Verification items for the finished model (mm, model axes). A direction names the side the tool comes from. Coordinates: 2 decimals unless noted, no trailing zeros. Loops run counter-clockwise (first coordinate to the right, second up) from the corner with the lowest first, then second, coordinate; pieces in that order, holes last. Notation, with made-up numbers: (48.25, -24.5) - (65.25, -24.5) arc R19 cw to (65.25, -18.5) - close; hole circle Ø10 at (1, 0.5). An arc over 180 degrees is marked (long way). One line per item, written item: value. Start each with the question number.
(1) Draft check along X on faces 5 (the face through (87, 3, 103.5)), 6 (the face through (-121.539, 3, -63)), 7 (the face through (-83, 3, -94.5)). Enter one of: +X half, -X half, draft (parallel to the pull), parting line (faces both ways), or undercut.
(2) Section check A-A (x = -71). Record the boundary of the cut face in (y, z), plus the area to 3 significant figures.
(3) Gauge pin test, flat ends, axial feed: P1, Ø1.8, axis at y = 2, z = -61, coming from the -X side; P2, Ø2, axis at x = -88.5, y = 3, coming from the +Z side. Record the tip position at first contact, or that the pin passes through.
(4) Set-up check for faces 1 (the face through (42.461, 3, -97)), 2 (the face through (96.461, 3, -80)), 3 (the face through (-82, 3, 97.5)), 4 (the face through (-121.539, 3, 29)): record each of +Z, -Z, +X, -X, +Y, -Y from which the full face is reachable in a straight line by a thin tool's end or side.
(5) Section check C-C (z = -68). Record the boundary of the cut face in (x, y).
(6) Section check B-B (y = 3.9). Count the separate pieces of the cut face and the enclosed holes in it, plus the area to 3 significant figures.
(7) Thickness scan on probe 1 along X at (y, z) = (2.1, 23); probe 2 along Z at (x, y) = (68.5, 5.25); probe 3 along X at (y, z) = (3.75, 42). Record the ranges inside material, lowest first. Write a range as [from, to].
Autodesk Inventor part; units mm, degrees
ref_plane "YZ Plane" through (0, 0, 0) normal (1, 0, 0) x (0, 1, 0)
ref_plane "XZ Plane" through (0, 0, 0) normal (0, 1, 0) x (-1, 0, 0)
ref_plane "XY Plane" through (0, 0, 0) normal (0, 0, 1) x (1, 0, 0)
sketch "Эскиз1" plane through (0, 0, 0) normal (0, 1, 0) x (-1, 0, 0)
  line L0 (127.5386, 103.5005) -> (-102.4614, 103.5005)
  line L1 (-102.4614, 103.5005) -> (-102.4614, -100.4995)
  line L2 (-102.4614, -100.4995) -> (127.5386, -100.4995)
  line L3 (127.5386, -100.4995) -> (127.5386, 103.5005)
  line L4 (127.5386, -100.4995) -> (97.5386, -100.4995)
  line L5 (97.5386, -100.4995) -> (97.5386, -94.4995)
  line L6 (97.5386, -94.4995) -> (127.5386, -94.4995)
  line L7 (127.5386, -94.4995) -> (127.5386, -100.4995)
  line L8 (97.5386, -94.4995) -> (67.5386, -94.4995)
  line L9 (67.5386, -94.4995) -> (67.5386, -100.4995)
  line L10 (67.5386, -100.4995) -> (97.5386, -100.4995)
  line L11 (97.5386, -100.4995) -> (97.5386, -94.4995)
  line L12 (6.9803, -100.4995) -> (67.5386, -100.4995)
  line L13 (67.5386, -100.4995) -> (67.5386, -94.4995)
  line L14 (-42.4614, -94.4995) -> (-42.4614, -100.4995)
  line L15 (-42.4614, -100.4995) -> (-2.4614, -100.4995)
  line L16 (-42.4614, -94.4995) -> (-72.4614, -94.4995)
  line L17 (-72.4614, -94.4995) -> (-72.4614, -100.4995)
  line L18 (-72.4614, -100.4995) -> (-42.4614, -100.4995)
  line L19 (-42.4614, -100.4995) -> (-42.4614, -94.4995)
  line L20 (-72.4614, -94.4995) -> (-102.4614, -94.4995)
  line L21 (-102.4614, -94.4995) -> (-102.4614, -100.4995)
  line L22 (-102.4614, -100.4995) -> (-72.4614, -100.4995)
  line L23 (-72.4614, -100.4995) -> (-72.4614, -94.4995)
  line L24 (-42.4614, -94.4995) -> (-2.4614, -94.4995)
  line L25 (-2.4614, -94.4995) -> (-2.4614, -100.4995)
  line L26 (-2.4614, -100.4995) -> (-42.4614, -100.4995)
  line L27 (-42.4614, -100.4995) -> (-42.4614, -94.4995)
  line L28 (-2.4614, -100.4995) -> (27.5386, -100.4995)
  line L29 (27.5386, -100.4995) -> (27.5386, -94.4995)
  line L30 (27.5386, -94.4995) -> (-2.4614, -94.4995)
  line L31 (-2.4614, -94.4995) -> (-2.4614, -100.4995)
  line L32 (67.5386, -94.4995) -> (27.5386, -94.4995)
  line L33 (27.5386, -94.4995) -> (27.5386, -100.4995)
  line L34 (27.5386, -100.4995) -> (67.5386, -100.4995)
  line L35 (67.5386, -100.4995) -> (67.5386, -94.4995)
  line L36 (-102.4614, 97.5005) -> (127.5386, 97.5005)
  line L37 (127.5386, 97.5005) -> (97.5386, 97.5005)
  line L38 (97.5386, 97.5005) -> (97.5386, 103.5005)
  line L39 (97.5386, 103.5005) -> (127.5386, 103.5005)
  line L40 (127.5386, 103.5005) -> (127.5386, 97.5005)
  line L41 (97.5386, 103.5005) -> (67.5386, 103.5005)
  line L42 (67.5386, 103.5005) -> (67.5386, 97.5005)
  line L43 (67.5386, 97.5005) -> (97.5386, 97.5005)
  line L44 (97.5386, 97.5005) -> (97.5386, 103.5005)
  line L45 (6.9803, 97.5005) -> (67.5386, 97.5005)
  line L46 (67.5386, 97.5005) -> (67.5386, 103.5005)
  line L47 (-42.4614, 103.5005) -> (-42.4614, 97.5005)
  line L48 (-42.4614, 97.5005) -> (-2.4614, 97.5005)
  line L49 (-42.4614, 103.5005) -> (-72.4614, 103.5005)
  line L50 (-72.4614, 103.5005) -> (-72.4614, 97.5005)
  line L51 (-72.4614, 97.5005) -> (-42.4614, 97.5005)
  line L52 (-42.4614, 97.5005) -> (-42.4614, 103.5005)
  line L53 (-72.4614, 103.5005) -> (-102.4614, 103.5005)
  line L54 (-102.4614, 103.5005) -> (-102.4614, 97.5005)
  line L55 (-102.4614, 97.5005) -> (-72.4614, 97.5005)
  line L56 (-72.4614, 97.5005) -> (-72.4614, 103.5005)
  line L57 (-42.4614, 103.5005) -> (-2.4614, 103.5005)
  line L58 (-2.4614, 103.5005) -> (-2.4614, 97.5005)
  line L59 (-2.4614, 97.5005) -> (-42.4614, 97.5005)
  line L60 (-42.4614, 97.5005) -> (-42.4614, 103.5005)
  line L61 (-2.4614, 97.5005) -> (27.5386, 97.5005)
  line L62 (27.5386, 97.5005) -> (27.5386, 103.5005)
  line L63 (27.5386, 103.5005) -> (-2.4614, 103.5005)
  line L64 (-2.4614, 103.5005) -> (-2.4614, 97.5005)
  line L65 (67.5386, 103.5005) -> (27.5386, 103.5005)
  line L66 (27.5386, 103.5005) -> (27.5386, 97.5005)
  line L67 (27.5386, 97.5005) -> (67.5386, 97.5005)
  line L68 (67.5386, 97.5005) -> (67.5386, 103.5005)
  line L69 (-102.4614, 63.5005) -> (-96.4614, 63.5005)
  line L70 (-96.4614, 63.5005) -> (-96.4614, 33.5005)
  line L71 (-96.4614, 33.5005) -> (-102.4614, 33.5005)
  line L72 (-102.4614, 33.5005) -> (-102.4614, 63.5005)
  line L73 (-102.4614, -30.4995) -> (-96.4614, -30.4995)
  line L74 (-96.4614, -30.4995) -> (-96.4614, -60.4995)
  line L75 (-96.4614, -60.4995) -> (-102.4614, -60.4995)
  line L76 (-102.4614, -60.4995) -> (-102.4614, -30.4995)
  line L77 (127.5386, 63.5005) -> (121.5386, 63.5005)
  line L78 (121.5386, 33.5005) -> (127.5386, 33.5005)
  line L79 (127.5386, 33.5005) -> (127.5386, 63.5005)
  line L80 (127.5386, -50.4995) -> (93.2543, -50.4995)
  line L81 (121.5386, -60.4995) -> (127.5386, -60.4995)
  line L82 (127.5386, -60.4995) -> (127.5386, -50.4995)
  line L83 (-102.4614, 88.5005) -> (-96.4614, 88.5005)
  line L84 (-96.4614, 88.5005) -> (-96.4614, 78.5005)
  line L85 (-96.4614, 78.5005) -> (-102.4614, 78.5005)
  line L86 (-102.4614, 78.5005) -> (-102.4614, 88.5005)
  line L87 (-102.4614, -75.4995) -> (-96.4614, -75.4995)
  line L88 (-96.4614, -75.4995) -> (-96.4614, -85.4995)
  line L89 (-96.4614, -85.4995) -> (-102.4614, -85.4995)
  line L90 (-102.4614, -85.4995) -> (-102.4614, -75.4995)
  line L91 (127.5386, 73.5005) -> (121.5386, 73.5005)
  line L92 (121.5386, 73.5005) -> (121.5386, 58.5005)
  line L93 (121.5386, 58.5005) -> (127.5386, 58.5005)
  line L94 (127.5386, 58.5005) -> (127.5386, 73.5005)
  line L95 (127.5386, -55.4995) -> (121.5386, -55.4995)
  line L96 (121.5386, -55.4995) -> (121.5386, -70.4995)
  line L97 (121.5386, -70.4995) -> (127.5386, -70.4995)
  line L98 (127.5386, -70.4995) -> (127.5386, -55.4995)
  line L99 (127.5386, 38.5005) -> (121.5386, 38.5005)
  line L100 (121.5386, 38.5005) -> (121.5386, 18.5005)
  line L101 (121.5386, 18.5005) -> (127.5386, 18.5005)
  line L102 (127.5386, 18.5005) -> (127.5386, 38.5005)
  line L103 (127.5386, -15.4995) -> (121.5386, -15.4995)
  line L104 (121.5386, -15.4995) -> (121.5386, -35.4995)
  line L105 (121.5386, -35.4995) -> (127.5386, -35.4995)
  line L106 (127.5386, -35.4995) -> (127.5386, -15.4995)
  point P0 (0, 0)
  point P1 (-42.4614, -97.4995)
  point P2 (67.5386, -97.4995)
  point P3 (-42.4614, 100.5005)
  point P4 (67.5386, 100.5005)
  point P5 (-99.4614, -60.4995)
  point P6 (97.5386, 103.5005)
  point P7 (67.5386, 103.5005)
  point P8 (27.5386, 103.5005)
  point P9 (27.5386, 97.5005)
  point P10 (-2.4614, 103.5005)
  point P11 (-42.4614, 103.5005)
  point P12 (-102.4614, 33.5005)
  point P13 (-2.4614, -100.4995)
  point P14 (124.5386, 63.5005)
  point P15 (124.5386, -60.4995)
  point P16 (127.5386, 33.5005)
  point P17 (127.5386, 97.5005)
  point P18 (-102.4614, 97.5005)
  point P19 (97.5386, 97.5005)
  point P20 (27.5386, 103.5005)
  point P21 (-2.4614, 97.5005)
  point P22 (27.5386, 97.5005)
  point P23 (-2.4614, -100.4995)
  point P24 (-99.4614, 88.5005)
  point P25 (-99.4614, 78.5005)
  point P26 (-99.4614, 63.5005)
  point P27 (-99.4614, -75.4995)
  point P28 (124.5386, 73.5005)
  point P29 (124.5386, 58.5005)
  point P30 (124.5386, -70.4995)
  point P31 (124.5386, 38.5005)
  point P32 (124.5386, -55.4995)
  point P33 (124.5386, -35.4995)
  dimension "d0" = 230
  dimension "d1" = 204
  dimension "d2" = 6
  dimension "d3" = 30
  dimension "d4" = 30
  dimension "d5" = 30
  dimension "d6" = 30
  dimension "d8" = 40
  dimension "d10" = 40
  dimension "d11" = 230
  dimension "d13" = 6
  dimension "d14" = 30
  dimension "d15" = 30
  dimension "d16" = 30
  dimension "d17" = 30
  dimension "d18" = 40
  dimension "d19" = 40
  dimension "d20" = 40
  dimension "d21" = 30
  dimension "d22" = 40
  dimension "d23" = 30
  dimension "d24" = 6
  dimension "d27" = 6
  dimension "d28" = 40
  dimension "d29" = 40
  dimension "d30" = 30
  dimension "d31" = 30
  dimension "d84" = 10
  dimension "d85" = 15
  dimension "d86" = 15
  dimension "d87" = 10
  dimension "d88" = 6
  dimension "d89" = 6
  dimension "d90" = 15
  dimension "d91" = 15
  dimension "d92" = 30
  dimension "d93" = 30
  dimension "d94" = 20
  dimension "d95" = 20
  dimension "d96" = 20
  dimension "d97" = 20
extrude "Выдавливание1" add sketch "Эскиз1" along normal blind 6 contours L3 L36 L38 L0 | L3 L91 L92 L93 L99 L100 L101 L103 L104 L105 L95 L96 L97 L6 L8 L32 L30 L24 L16 L20 L1 L89 L88 L87 L75 L74 L73 L71 L70 L69 L85 L84 L83 L36 | L42 L36 L62 L0 | L58 L36 L47 L0 | L50 L36 L1 L0 | L3 L2 L5 L6 | L9 L2 L29 L32 | L20 L17 L2 L1 | L25 L2 L14 L24
sketch "Эскиз2" plane through (0, 6, 0) normal (0, 1, 0) x (1, 0, 0)
  point P0 (0, 0)
sketch "Эскиз5" plane through (0, 0, 0) normal (0, -1, 0) x (1, 0, 0)
  circle A0 centre (22.4614, 100.5005) radius 1.5
  circle A1 centre (-47.5386, 100.5005) radius 1.5
  circle A2 centre (-47.5386, -97.4995) radius 1.5
  circle A3 centre (22.4614, -97.4995) radius 1.5
  line L0 (42.4614, -100.4995) -> (2.4614, -100.4995)
  line L1 (-27.5386, -100.4995) -> (-67.5386, -100.4995)
  line L2 (42.4614, -94.4995) -> (42.4614, -100.4995)
  line L3 (-27.5386, -94.4995) -> (-27.5386, -100.4995)
  line L4 (2.4614, 103.5005) -> (42.4614, 103.5005)
  line L5 (-67.5386, 103.5005) -> (-27.5386, 103.5005)
  line L6 (2.4614, 97.5005) -> (2.4614, 103.5005)
  line L7 (-27.5386, 103.5005) -> (-27.5386, 97.5005)
  point P0 (0, 0)
  point P1 (42.4614, -97.4995)
  point P2 (2.4614, 100.5005)
  dimension "d41" = 3
  dimension "d42" = 3
  dimension "d43" = 3
  dimension "d44" = 20
  dimension "d45" = 20
  dimension "d46" = 3
  dimension "d47" = 3
  dimension "d48" = 20
  dimension "d49" = 20
extrude "Выдавливание3" cut sketch "Эскиз5" against normal through all
sketch "Эскиз6" plane through (0, 6, 0) normal (0, 1, 0) x (1, 0, 0)
  line L0 (76.6943, 94.4995) -> (62.6943, 94.4995)
  line L1 (62.2284, -103.5005) -> (76.2284, -103.5005)
  circle A0 centre (79.2284, -83.5005) radius 1.5
  circle A1 centre (59.2284, -83.5005) radius 1.5
  circle A2 centre (79.2284, -63.5005) radius 1.5
  circle A3 centre (59.2284, -63.5005) radius 1.5
  line L2 (79.2284, -159.6407) -> (79.2284, -82.1128) construction
  point P0 (0, 0)
  dimension "d52" = 3
  dimension "d53" = 20
  dimension "d54" = 20
  dimension "d55" = 20
  dimension "d56" = 20
  dimension "d57" = 20
  dimension "d58" = 20
  dimension "d59" = 3
extrude "Выдавливание4" cut sketch "Эскиз6" against normal through all
ref_plane "РабПлоскость1" through (42.4614, 0, 1.5005) normal (0, 0, -1) x (-1, 0, 0)
mirror "Зеркальное отражение1" about plane through (42.4614, 0, 1.5005) normal (0, 0, -1) of "Выдавливание4"
sketch "Эскиз7" plane through (0, 0, 0) normal (0, -1, 0) x (1, 0, 0)
  line L0 (96.4614, -60.4995) -> (96.4614, -30.4995)
  line L1 (96.4614, -30.4995) -> (102.4614, -30.4995)
  line L2 (102.4614, -30.4995) -> (102.4614, -60.4995)
  line L3 (102.4614, -60.4995) -> (96.4614, -60.4995)
  line L4 (96.4614, 39.5005) -> (96.4614, 69.5005)
  line L5 (96.4614, 69.5005) -> (102.4614, 69.5005)
  line L6 (102.4614, 69.5005) -> (102.4614, 33.5005)
  line L7 (102.4614, 39.5005) -> (96.4614, 39.5005)
  line L8 (102.4614, 13.4114) -> (96.4614, 13.4114)
  line L9 (96.4614, 16.4114) -> (102.4614, 16.4114)
  line L10 (96.4614, -6.5886) -> (102.4614, -6.5886)
  line L11 (102.4614, -9.5886) -> (96.4614, -9.5886)
  circle A0 centre (99.4614, 14.9114) radius 1.5
  circle A1 centre (99.4614, -8.0886) radius 1.5
  line L12 (102.4614, 33.5005) -> (102.4614, -30.4995)
  point P0 (0, 0)
  point P1 (99.4614, 13.4114)
  dimension "d62" = 3
  dimension "d63" = 3
  dimension "d64" = 3
  dimension "d65" = 3
  dimension "d66" = 1.5
  dimension "d67" = 1.5
extrude "Выдавливание5" cut sketch "Эскиз7" against normal blind 6 contours A1 | A0
sketch "Эскиз9" plane through (0, 0, 0) normal (0, -1, 0) x (1, 0, 0)
  circle A0 centre (-42.5386, 27.5005) radius 1.5
  circle A1 centre (-42.6205, -30.4995) radius 1.5
  circle A2 centre (-97.5386, -27.4995) radius 1.5
  circle A3 centre (-97.5386, 27.5005) radius 1.5
  line L0 (-127.5386, -100.4995) -> (-127.5386, 103.5005)
  line L1 (-97.5386, 97.5005) -> (-67.5386, 97.5005)
  line L2 (-27.5386, 97.5005) -> (2.4614, 97.5005)
  point P0 (0, 0)
  dimension "d70" = 3
  dimension "d71" = 3
  dimension "d72" = 3
  dimension "d73" = 3
  dimension "d74" = 55
  dimension "d75" = 52
  dimension "d76" = 55
  dimension "d77" = 52
  dimension "d78" = 30
  dimension "d79" = 30
  dimension "d80" = 70
  dimension "d81" = 70
extrude "Выдавливание6" cut sketch "Эскиз9" against normal up to surface (6 mm away)
sketch "Эскиз10" plane through (0, 0, 0) normal (0, -1, 0) x (1, 0, 0)
  circle A0 centre (-124.5386, 48.5005) radius 1.5
  circle A1 centre (-124.5386, 1.5005) radius 1.5
  circle A2 centre (-124.5386, -45.4995) radius 1.5
  line L0 (-127.5386, -35.4995) -> (-121.5386, -35.4995)
  line L1 (-127.5386, -55.4995) -> (-127.5386, -35.4995)
  line L2 (-127.5386, 38.5005) -> (-127.5386, 58.5005)
  line L3 (-121.5386, 38.5005) -> (-127.5386, 38.5005)
  line L4 (-127.5386, 18.5005) -> (-121.5386, 18.5005)
  line L5 (-127.5386, -15.4995) -> (-127.5386, 18.5005)
  point P0 (0, 0)
  point P1 (-124.5386, -35.4995)
  point P2 (-127.5386, 48.5005)
  point P3 (-124.5386, 18.5005)
  dimension "d98" = 3
  dimension "d99" = 3
  dimension "d100" = 3
  dimension "d101" = 10
  dimension "d102" = 3
  dimension "d103" = 3
  dimension "d104" = 10
  dimension "d105" = 17
  dimension "d106" = 3
extrude "Выдавливание7" cut sketch "Эскиз10" against normal blind 6
properties part number "Низ робота"
Responses:
1. face 5: draft
1. face 6: -X half
1. face 7: undercut
2. outline: (0, -94.5) - (6, -94.5) - (6, 97.5) - (0, 97.5) - close
2. area: 1,150 mm²
3. P1: stops at x = -121.54
3. P2: stops at z = 97.5
4. face 1: -Z, +Y, -Y
4. face 2: +X, +Y, -Y
4. face 3: +Z, +Y, -Y
4. face 4: -X, +Y, -Y
5. outline: (-121.54, 0) - (102.46, 0) - (102.46, 6) - (-121.54, 6) - close
6. separate pieces: 1
6. enclosed holes: 21
6. area: 44,800 mm²
7. probe 1: x = [-121.54, 102.46]
7. probe 2: z = [-94.5, 97.5]
7. probe 3: x = [-127.54, 96.46]
